Input: part model. Units: mm. Frame: model coordinates. A direction names the side the tool comes from. Give positions to 0.01 mm unless a question says otherwise; leave off trailing zeros. Write each loop counter-clockwise with the first axis right and the second up, starting at its lowest first coordinate (ties: lowest second). Pieces come first, ordered by that corner, then holes.
```python
from build123d import *

# Parameters (mm, degrees)
F0_R     = 50.8
F1_DEPTH = 38.1
F2_R     = 31.75
F3_DEPTH = 25.4
F4_R     = 3.175
F5_DEPTH = 6.35
F6_R     = 5.08


with BuildPart() as f1:
    # F0 (on Top) → F1 (new body)
    with BuildSketch(Plane.XY):
        Circle(F0_R)
    extrude(amount=F1_DEPTH)

    # F2 (on face) → F3 (join)
    with BuildSketch(Plane.XY.offset(38.1)):
        Circle(F2_R)
    extrude(amount=F3_DEPTH)

    # F4 (on face) → F5 (cut)
    with BuildSketch(Plane.XY.offset(63.5)):
        with Locations((-17.392001, 0)):
            Circle(F4_R)
        with Locations((0, -17.392001)):
            Circle(F4_R)
        with Locations((17.392001, 0)):
            Circle(F4_R)
        with Locations((0, 17.392001)):
            Circle(F4_R)
        Circle(F4_R)
    extrude(amount=-F5_DEPTH, mode=Mode.SUBTRACT)

    # F6
    f6_edges = [f1.edges().sort_by_distance(p)[0] for p in [
        (-31.75, 0, 63.5),
        (-50.8, 0, 38.1),
    ]]
    fillet(f6_edges, radius=F6_R)


solid = f1.part
```
Q1. Section A-A, the plane x = 0. Return the cut outline in (y, z) (3 decimals), then the cut area to 3 significant figures.
Q2. Mould query, pull axis Y, two halves, no side actions, for faces 1 (the flat face through (-1, 1, 0)), 2 (the flat face through (0, 0, 57.15)), 3 (the cylindrical face through (-11.012, -49.592, 16.279)). Classes: +Y half, -Y half, draft (parallel to the pull), parting line (faces both ways), or undercut.
Q3. Access query for faces 4 (the flat face through (0, -6, 63.5)), 5 (the flat face through (0, 17, 57.15)). Directions: +Z, -Z, +X, -X, +Y, -Y. A direction counts if a zero-diameter tool reaches every point of the face in a straight line with its end or side. Return the directions, or none.
Q4. Material intervals for line 1 along Y through (x, z) = (0, 61) (3 decimals); line 2 along Y through (x, z) = (0, 59) (3 decimals); line 3 along Z through (x, y) = (-5, -40.5), sorted ascending.
Q5. Pin query (flat end, axial travel): pin 1 (7 mm diameter, centred on x = 18, y = 1, fed in from +Z); pin 2 (1 mm diameter, centred on y = -1.5, z = 44, fed in from -X); pin 3 (5.5 mm diameter, centred on x = 17.39, y = 0, fed in from +Z); pin 4 (8 mm diameter, centred on x = -27, y = 30, fed in from +Z). Return the tip coordinate at first contact, or that it passes through.
Q6. Section C-C, the plane z = 12. Return the cut outline in (x, y), then the cut area to 3 significant figures.
Solutions:
1. outline: (-50.8, 0) - (50.8, 0) - (50.8, 33.02) arc R5.08 ccw to (45.72, 38.1) - (31.75, 38.1) - (31.75, 58.42) arc R5.08 ccw to (26.67, 63.5) - (20.567, 63.5) - (20.567, 57.15) - (14.217, 57.15) - (14.217, 63.5) - (3.175, 63.5) - (3.175, 57.15) - (-3.175, 57.15) - (-3.175, 63.5) - (-14.217, 63.5) - (-14.217, 57.15) - (-20.567, 57.15) - (-20.567, 63.5) - (-26.67, 63.5) arc R5.08 ccw to (-31.75, 58.42) - (-31.75, 38.1) - (-45.72, 38.1) arc R5.08 ccw to (-50.8, 33.02) - close
1. area: 5,340 mm2
2. face 1: draft
2. face 2: undercut
2. face 3: parting line
3. face 4: +Z, +X, -X, +Y, -Y
3. face 5: +Z
4. line 1: y = -31.046 to -20.567, -14.217 to -3.175, 3.175 to 14.217, 20.567 to 31.046
4. line 2: y = -31.717 to -20.567, -14.217 to -3.175, 3.175 to 14.217, 20.567 to 31.717
4. line 3: z = 0 to 38.1
5. pin 1: stops at z = 63.5
5. pin 2: stops at x = -31.73
5. pin 3: stops at z = 57.15
5. pin 4: stops at z = 38.1
6. outline: circle Ø101.6 at (0, 0)
6. area: 8,110 mm2
